```python
from build123d import *

# Parameters (mm, degrees)
SKETCH1_W                = 16.31
SKETCH1_H                = 5
BOSS_EXTRUDE3_DEPTH      = 5
CUT_EXTRUDE9_DEPTH       = 5
SKETCH4_R                = 1.4
CUT_EXTRUDE10_DEPTH      = 2.5
CUT_EXTRUDE10_DEPTH_BACK = 2.5


with BuildPart() as part:
    # Sketch1 → Boss-Extrude3 (new body)
    with BuildSketch(Plane.XY):
        Rectangle(SKETCH1_W, SKETCH1_H)
    extrude(amount=-BOSS_EXTRUDE3_DEPTH)

    # Sketch3 → Cut-Extrude9 (cut)
    with BuildSketch(Plane.XY):
        with BuildLine():
            Line((-3.355, -2.5), (3.355, -2.5))
            ThreePointArc((3.355, -2.5), (0, 0.855), (-3.355, -2.5))
        make_face()
    extrude(amount=-CUT_EXTRUDE9_DEPTH, mode=Mode.SUBTRACT)

    # Sketch4 → Cut-Extrude10 (cut, two sides)
    with BuildSketch(Plane(origin=(0, 0, 0), x_dir=(1, 0, 0), z_dir=(0, 1, 0))) as cut_extrude10_sk:
        with Locations((-5.755, 2.5)):
            Circle(SKETCH4_R)
        with Locations((5.755, 2.5)):
            Circle(SKETCH4_R)
    extrude(amount=CUT_EXTRUDE10_DEPTH, mode=Mode.SUBTRACT)
    extrude(cut_extrude10_sk.sketch, amount=-CUT_EXTRUDE10_DEPTH_BACK, mode=Mode.SUBTRACT)


solid = part.part
```
Can you work these out from the model? Positions are in its coordinate system, mm. Give positions to 0.01 mm unless a question says otherwise; leave off trailing zeros. Loops run counter-clockwise (first coordinate to the right, second up) from the corner with the lowest first, then second, coordinate; pieces in that order, holes last. Notation, with made-up numbers: M -3,41.5 L 42,41.5 A20 ccw 42,70.5 Z; hole C -30,-13.75 d6. An arc over 180 degrees is marked long. Use CSV: the item, a comma, the result in double quotes. Start each with the question number.
1. If we mould it in two halves opening along X, with no side actions, what happens to faces 1 (the face through (0.074, 0.854, -2.465)), 2 (the face through (-0.1, 1.1, -5)), 3 (the face through (8.155, 0, -2))? For each: released by +X, released by -X, zero draft, split by the parting line, or undercut.
2. Imagine slicing it at C-C, the plane y = 2.1. Write out the boundary of the cut face in (x, z) (3 decimals), plus the area to 3 significant figures.
3. Imagine slicing it at A-A, the plane z = -2.5. Write out the boundary of the cut face in (x, y) (3 decimals), plus the area to 3 significant figures.
4. Imagine slicing it at D-D, the plane x = -7. Write out the boundary of the cut face in (y, z).
5. Imagine slicing it at B-B, the plane y = -0.95. Write out the boundary of the cut face in (x, z) (3 decimals).
6. For P1, Ø2, axis at x = -5.755, z = -2.5, coming from the +Y side, with a flat end and sliding along its axis, tell me the tip position at first contact or that it passes through.
7. If I drill on L1, parallel to X at y = 1.3, z = -2.5 (3 decimals); L2, parallel to X at y = -0.9, z = -2.5 (3 decimals); L3, parallel to X at y = 2.25, z = -1.75 (3 decimals), over which ranges is the centre line in solid material (lowest first)?
Response values:
1,face 1,"undercut"
1,face 2,"zero draft"
1,face 3,"released by +X"
2,outline,"M -8.155,-5 L 8.155,-5 L 8.155,0 L -8.155,0 Z; hole C -5.755,-2.5 d2.8; hole C 5.755,-2.5 d2.8"
2,area,"69.2 mm^2"
3,outline,"M -8.155,-2.5 L -7.155,-2.5 L -7.155,2.5 L -8.155,2.5 Z; M -4.355,-2.5 L -3.355,-2.5 A3.355 cw 3.355,-2.5 L 4.355,-2.5 L 4.355,2.5 L -4.355,2.5 Z; M 7.155,-2.5 L 8.155,-2.5 L 8.155,2.5 L 7.155,2.5 Z"
3,area,"35.9 mm^2"
4,outline,"M -2.5,-5 L 2.5,-5 L 2.5,-3.14 L -2.5,-3.14 Z; M -2.5,-1.86 L 2.5,-1.86 L 2.5,0 L -2.5,0 Z"
5,outline,"M -8.155,-5 L -2.975,-5 L -2.975,0 L -8.155,0 Z; M 2.975,-5 L 8.155,-5 L 8.155,0 L 2.975,0 Z; hole C -5.755,-2.5 d2.8; hole C 5.755,-2.5 d2.8"
6,P1,"through"
7,L1,"-8.155 to -7.155, -4.355 to 4.355, 7.155 to 8.155"
7,L2,"-8.155 to -7.155, -4.355 to -2.949, 2.949 to 4.355, 7.155 to 8.155"
7,L3,"-8.155 to -6.937, -4.573 to 4.573, 6.937 to 8.155"
